```python
from build123d import *

# Parameters (mm, degrees)
SKETCH1_W           = 7
SKETCH1_H           = 7
BOSS_EXTRUDE1_DEPTH = 3
CUT_EXTRUDE1_DEPTH  = 0.8


with BuildPart() as part:
    # Sketch1 → Boss-Extrude1 (new body)
    with BuildSketch(Plane(origin=(0, 0, 0), x_dir=(1, 0, 0), z_dir=(0, 1, 0))):
        Rectangle(SKETCH1_W, SKETCH1_H)
    extrude(amount=BOSS_EXTRUDE1_DEPTH)

    # Sketch2 → Cut-Extrude1 (cut)
    with BuildSketch(Plane(origin=(0, 3, 0), x_dir=(1, 0, 0), z_dir=(0, 1, 0))):
        with BuildLine():
            Line((-1.5, 2.5), (1.5, 2.5))
            ThreePointArc((1.5, 2.5), (2.207106781, 2.207106781), (2.5, 1.5))
            Line((2.5, 1.5), (2.5, -1.5))
            ThreePointArc((2.5, -1.5), (2.207106781, -2.207106781), (1.5, -2.5))
            Line((1.5, -2.5), (-1.5, -2.5))
            ThreePointArc((-1.5, -2.5), (-2.207106781, -2.207106781), (-2.5, -1.5))
            Line((-2.5, -1.5), (-2.5, 1.5))
            ThreePointArc((-2.5, 1.5), (-2.207106781, 2.207106781), (-1.5, 2.5))
        make_face()
    extrude(amount=-CUT_EXTRUDE1_DEPTH, mode=Mode.SUBTRACT)


solid = part.part
```
Verification items for the finished model (mm, model axes). A direction names the side the tool comes from. Round coordinates to 2 decimals unless told otherwise and drop trailing zeros. Loops run counter-clockwise (first coordinate to the right, second up) from the corner with the lowest first, then second, coordinate; pieces in that order, holes last. Notation, with made-up numbers: (-8, 11) -> (-3, 11) arc R5 ccw to (-3, 20) -> close; hole circle Ø2 at (59, 4). An arc over 180 degrees is marked (long way). Answer as a JSON object with one key per item and string values.
Q1. Section check A-A (y = 2.8). Record the boundary of the cut face in (x, z), then the cut area to 3 significant figures.
Data:
{"outline": "(-3.5, -3.5) -> (3.5, -3.5) -> (3.5, 3.5) -> (-3.5, 3.5) -> close; hole (-2.5, -1.5) arc R1 ccw to (-1.5, -2.5) -> (1.5, -2.5) arc R1 ccw to (2.5, -1.5) -> (2.5, 1.5) arc R1 ccw to (1.5, 2.5) -> (-1.5, 2.5) arc R1 ccw to (-2.5, 1.5) -> close", "area": "24.9 mm2"}
Q2. Draft check along Z on faces 3 (the flat face through (0, 1, 3.5)), 4 (the flat face through (-3.5, 1, 0)), 5 (the cylindrical face through (-2.215, 2.606, -2.199)). Enter one of: pulls with the +Z half, pulls with the -Z half, needs draft (parallel to the pull), parting line crosses it, or undercut.
Data:
{"face 3": "pulls with the +Z half", "face 4": "needs draft", "face 5": "undercut"}
Q3. Access from +Z, -Z, +X, -X, +Y, -Y to the whole of each face (thin tool, end or side, straight path). Record for faces 1 (the flat face through (0, 1, -3.5)), 2 (the cylindrical face through (-2.199, 2.606, 2.215)).
Data:
{"face 1": "-Z, +X, -X, +Y, -Y", "face 2": "+Y"}
Q4. Scan lines: line 1 (Z direction, x = -1.5, y = 2.6); line 2 (Y direction, x = -1, z = 1). Record each from-to range of solid material in increasing order. Write a range as from..to.
Data:
{"line 1": "z = -3.5..-2.5, 2.5..3.5", "line 2": "y = 0..2.2"}
Q5. Section check B-B (x = 0.5). Record the boundary of the cut face in (y, z), then the cut area to 3 significant figures.
Data:
{"outline": "(0, -3.5) -> (3, -3.5) -> (3, -2.5) -> (2.2, -2.5) -> (2.2, 2.5) -> (3, 2.5) -> (3, 3.5) -> (0, 3.5) -> close", "area": "17.0 mm2"}
Q6. Section check C-C (z = -0.5). Record the boundary of the cut face in (x, y), then the cut area to 3 significant figures.
Data:
{"outline": "(-3.5, 0) -> (3.5, 0) -> (3.5, 3) -> (2.5, 3) -> (2.5, 2.2) -> (-2.5, 2.2) -> (-2.5, 3) -> (-3.5, 3) -> close", "area": "17.0 mm2"}
